Geometry: final body of the model. Coordinates: model frame, mm. A direction names the side the tool comes from. Coordinates: 2 decimals unless noted, no trailing zeros. Write each loop counter-clockwise with the first axis right and the second up, starting at its lowest first coordinate (ties: lowest second). Pieces come first, ordered by that corner, then holes. Notation, with made-up numbers: (21, 52) -> (76, 52) arc R34 cw to (76, 88) -> close; hole circle Ø10 at (26.25, 58). An arc over 180 degrees is marked (long way). One line per item, written item: value. Start each with the question number.
from build123d import *

# Parameters (mm, degrees)
F0_R     = 12.7
F1_DEPTH = 6.35
F3_DEPTH = 38.1


with BuildPart() as f1:
    # F0 (on Front) → F1 (new body)
    with BuildSketch(Plane.XZ):
        Circle(F0_R)
    extrude(amount=F1_DEPTH)

    # F2 (on face) → F3 (join)
    with BuildSketch(Plane.XZ.offset(6.35)):
        Polygon((0, -8.441441), (8.441441, 0), (0, 8.441441), (-8.441441, 0), align=None)
    extrude(amount=F3_DEPTH)


solid = f1.part
Q1. Cut plane C-C on y = -22. Output: boundary loops of the cut face in (x, z), and give its area (3 significant figures).
Q2. Cut plane A-A on x = -2.5. Output: boundary loops of the cut face in (y, z).
Q3. Cut plane D-D on x = -9.75. Output: boundary loops of the cut face in (y, z).
Q4. First-contact query: P1, Ø3, axis at x = 3.5, z = -9, coming from the -Y side; P2, Ø8, axis at x = 9, y = -18.5, coming from the -Z side; P3, Ø8, axis at x = -3, y = -22, coming from the +Z side; P4, Ø1.5, axis at y = -12.5, z = 10, coming from the -X side. Flat tips, straight axial feed; report the tip coordinate or a pass-through.
Q5. Cut plane B-B on z = -6.75. Output: boundary loops of the cut face in (x, y).
Q6. Access query for faces 1 (the flat face through (3, -6.35, 6)), 2 (the flat face through (-4.16, -25.13, 4.28)), 3 (the flat face through (-4.28, -25.13, -4.16)), 4 (the flat face through (4.28, -25.13, 4.16)), 5 (the flat face through (4.16, -25.13, -4.28)). Directions: +Z, -Z, +X, -X, +Y, -Y. A direction counts if a zero-diameter tool reaches every point of the face in a straight line with its end or side. Return the directions, or none.
Q7. Line query: L1, parallel to Y at x = 5, z = 4; L2, parallel to Z at x = 2.5, y = -32.5; L3, parallel to X at y = -24.5, z = 4.75. Output: solid intervals per line, ascending. Write a range as from..to.
Solution:
1. outline: (-8.44, 0) -> (0, -8.44) -> (8.44, 0) -> (0, 8.44) -> close
1. area: 143 mm²
2. outline: (-44.45, -5.94) -> (-6.35, -5.94) -> (-6.35, -12.45) -> (0, -12.45) -> (0, 12.45) -> (-6.35, 12.45) -> (-6.35, 5.94) -> (-44.45, 5.94) -> close
3. outline: (-6.35, -8.14) -> (0, -8.14) -> (0, 8.14) -> (-6.35, 8.14) -> close
4. P1: y = -6.35
4. P2: z = -3.44
4. P3: z = 8.44
4. P4: through
5. outline: (-10.76, -6.35) -> (-1.69, -6.35) -> (-1.69, -44.45) -> (1.69, -44.45) -> (1.69, -6.35) -> (10.76, -6.35) -> (10.76, 0) -> (-10.76, 0) -> close
6. face 1: -Y
6. face 2: +Z, -X, -Y
6. face 3: -Z, -X, -Y
6. face 4: +Z, +X, -Y
6. face 5: -Z, +X, -Y
7. L1: -6.35..0
7. L2: -5.94..5.94
7. L3: -3.69..3.69
